from build123d import *

# Parameters (mm, degrees)
SKIZZE1_W                       = 13
SKIZZE1_H                       = 33
AUFSATZ_LINEAR_AUSTRAGEN1_DEPTH = 27.5
SKIZZE2_R                       = 5
AUFSATZ_LINEAR_AUSTRAGEN2_DEPTH = 10


with BuildPart() as part:
    # Skizze1 → Aufsatz-Linear austragen1 (new body)
    with BuildSketch(Plane(origin=(0, 0, 0), x_dir=(1, 0, 0), z_dir=(0, 1, 0))):
        with Locations((-7.102941176, -3.558823529)):
            Rectangle(SKIZZE1_W, SKIZZE1_H)
    extrude(amount=AUFSATZ_LINEAR_AUSTRAGEN1_DEPTH)

    # Skizze2 → Aufsatz-Linear austragen2 (add)
    with BuildSketch(Plane(origin=(0, 0, 0), x_dir=(1, 0, 0), z_dir=(0, 1, 0))):
        with Locations((-7.102941176, -3.558823529)):
            Circle(SKIZZE2_R)
    extrude(amount=-AUFSATZ_LINEAR_AUSTRAGEN2_DEPTH)


solid = part.part
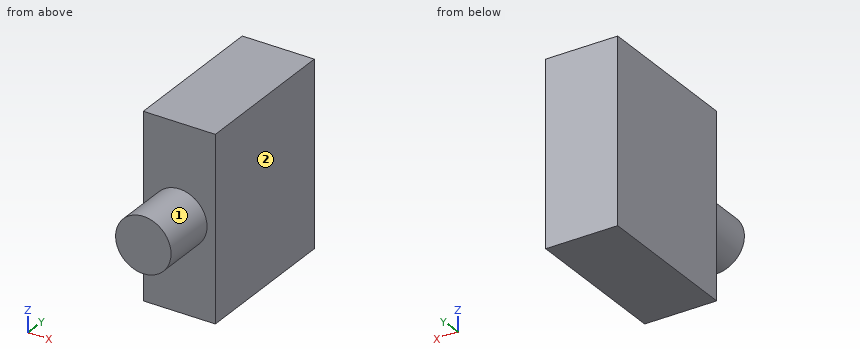
Work out the finished part from the listing and answer in its coordinate system (mm). Face numbers are marked on the shaded views. A direction names the side the tool comes from. Round coordinates to 2 decimals unless told otherwise and drop trailing zeros. Write each loop counter-clockwise with the first axis right and the second up, starting at its lowest first coordinate (ties: lowest second). Pieces come first, ordered by that corner, then holes. Notation, with made-up numbers: (7.5, 8.25) -> (12.5, 8.25) arc R15 cw to (12.5, 16.25) -> close; hole circle Ø1 at (85, 73). An arc over 180 degrees is marked (long way). Write each question's results on one line, items separated by ' | '.
Item 1: A cutting plane is placed at C-C, the plane y = -0.5. Determine the outline of the cut face in (x, z), plus the area to 3 significant figures.
Result set:
outline: circle Ø10 at (-7.1, 3.56) | area: 78.5 mm^2
Item 2: Find the intervals of material crossed by line 1 along Y through (x, z) = (-12.5, -6.5); line 2 along Z through (x, y) = (-7, -7); line 3 along Z through (x, y) = (-4.75, -8), in increasing order. Write a range as [from, to].
Result set:
line 1: [0, 27.5] | line 2: [-1.44, 8.56] | line 3: [-0.85, 7.97]
Item 3: Which of the six approach directions +Z, -Z, +X, -X, +Y, -Y give full straight-line access (tool end or side, diameter ignored) to the marked faces 1 and 2?
Result set:
face 1: -Y | face 2: +Z, -Z, +X, +Y, -Y
Item 4: A cutting plane is placed at B-B, the plane z = 4. Determine the outline of the cut face in (x, y), plus the area to 3 significant figures.
Result set:
outline: (-13.6, 0) -> (-12.08, 0) -> (-12.08, -10) -> (-2.12, -10) -> (-2.12, 0) -> (-0.6, 0) -> (-0.6, 27.5) -> (-13.6, 27.5) -> close | area: 457 mm^2
Item 5: A cutting plane is placed at D-D, the plane z = -6.5. Determine the outline of the cut face in (x, y), plus the area to 4 significant figures.
Result set:
outline: (-13.6, 0) -> (-0.6, 0) -> (-0.6, 27.5) -> (-13.6, 27.5) -> close | area: 357.5 mm^2
Item 6: Flat-ended cylindrical pins translate along their axes: P1, Ø1, axis at x = -12, y = -3.5, coming from the -Z side; P2, Ø4, axis at x = -6.5, z = 12.5, coming from the -Y side; P3, Ø6.5, axis at x = -9.5, z = -4, coming from the -Y side. Find the tip coordinate at first contact, or state that the pin passes through.
Result set:
P1: z = 1.18 | P2: y = 0 | P3: y = -10
Item 7: A cutting plane is placed at A-A, the plane x = -5.5. Determine the outline of the cut face in (y, z), plus the area to 3 significant figures.
Result set:
outline: (-10, -1.18) -> (0, -1.18) -> (0, -12.94) -> (27.5, -12.94) -> (27.5, 20.06) -> (0, 20.06) -> (0, 8.29) -> (-10, 8.29) -> close | area: 1,000 mm^2
